```python
from build123d import *

# Parameters (mm, degrees)
SKETCH_1_W         = 25.5
SKETCH_1_H         = 25
EXTRUDE_1_DEPTH    = 4
SKETCH_6_W         = 25.5
SKETCH_6_H         = 7
EXTRUDE_2_DEPTH    = 9
HOLE_WIZARD_M3_1_D = 2.5
HOLE_WIZARD_M4_3_D = 3.3
FILLET_1_R         = 1


with BuildPart() as part:
    # 草图1 → 凸台-拉伸1 (new body)
    with BuildSketch(Plane(origin=(0, 0, 0), x_dir=(1, 0, 0), z_dir=(0, 1, 0))):
        Rectangle(SKETCH_1_W, SKETCH_1_H)
    extrude(amount=EXTRUDE_1_DEPTH)

    # 草图6 → 凸台-拉伸2 (add)
    with BuildSketch(Plane(origin=(0, 4, 0), x_dir=(1, 0, 0), z_dir=(0, 1, 0))):
        with Locations((0, 9)):
            Rectangle(SKETCH_6_W, SKETCH_6_H)
        with Locations((0, -9)):
            Rectangle(SKETCH_6_W, SKETCH_6_H)
    extrude(amount=EXTRUDE_2_DEPTH)

    # M3 螺纹孔1 (through all)
    with Locations(Plane(origin=(6.35, 0, 0), x_dir=(0, 0, -1), z_dir=(0, -1, 0))):
        with Locations((0, 0), (0, -12.7)):
            Hole(HOLE_WIZARD_M3_1_D / 2)

    # M4 螺纹孔3 (through all)
    with Locations(Plane(origin=(7.5, 0, 8.5), x_dir=(0, 0, -1), z_dir=(0, -1, 0))):
        with Locations((0, 0), (0, -15), (17, -15), (17, 0)):
            Hole(HOLE_WIZARD_M4_3_D / 2)

    # 圆角1
    fillet_1_edges = [part.edges().sort_by_distance(p)[0] for p in [
        (0, 4, -5.5),
        (0, 13, -12.5),
        (0, 4, 5.5),
        (0, 13, 12.5),
        (0, 0, 12.5),
        (0, 0, -12.5),
    ]]
    fillet(fillet_1_edges, radius=FILLET_1_R)


solid = part.part
```
Check sheet for the modelled part. Datum: model origin and axes. Units: mm. A direction names the side the tool comes from. Coordinates: 2 decimals unless noted, no trailing zeros. Write each loop counter-clockwise with the first axis right and the second up, starting at its lowest first coordinate (ties: lowest second). Pieces come first, ordered by that corner, then holes. Notation, with made-up numbers: M -37,-10 L -3,-10 A26 cw -3,25 Z; hole C 17,46 d5. An arc over 180 degrees is marked long. Write item = value, one per line. Start each with the question number.
1. Sectioned sample at C-C (x = -6.35). Record the cut outline in (y, z), then the cut area to 3 significant figures.
2. Sectioned sample at D-D (x = 0). Record the cut outline in (y, z), then the cut area to 3 significant figures.
3. Thickness scan on probe 1 along X at (y, z) = (10, 8.5); probe 2 along X at (y, z) = (10.25, -9.25); probe 3 along Z at (x, y) = (1, 6). Record the ranges inside material, lowest first.
4. Sectioned sample at A-A (y = 8.5). Record the cut outline in (x, z).
5. Go/stop test with flat-tipped pins: pin 1 (2.5 mm diameter, centred on x = -2, z = -2, fed in from +Y); pin 2 (3 mm diameter, centred on x = 6.35, z = 0, fed in from -Y). Record where each tip stops, or that it passes through.
6. Mould release check, pull along X, two halves, no side actions. Record for faces 1 (the flat face through (-12.75, 3.5, 0.2)), 2 (the cylindrical face through (-5.11, 2.03, -0.16)), 3 (the cylindrical face through (-7.43, 6.59, -10.15)), 4 (the flat face through (0, 6, 12.5)): pulls with the +X half, pulls with the -X half, needs draft (parallel to the pull), parting line crosses it, or undercut.
7. Sectioned sample at B-B (z = -0.75). Record the cut outline in (x, y), then the cut area to 3 significant figures.
8. Tool access check on faces 5 (the cylindrical face through (7.59, 2.03, -0.16)), 6 (the flat face through (0, 9, 5.5)). Record the directions out of +Z, -Z, +X, -X, +Y, -Y that give a thin tool (end or side, any length) a straight path to the whole face; none if there is none.
The answers:
q1.outline = M 0,-11.5 A1 ccw 1,-12.5 L 12,-12.5 A1 ccw 13,-11.5 L 13,-9.68 L 0,-9.68 Z; M 0,-7.32 L 13,-7.32 L 13,-5.5 L 5,-5.5 A1 cw 4,-4.5 L 4,-1.25 L 0,-1.25 Z; M 0,1.25 L 4,1.25 L 4,4.5 A1 cw 5,5.5 L 13,5.5 L 13,7.32 L 0,7.32 Z; M 0,9.68 L 13,9.68 L 13,11.5 A1 ccw 12,12.5 L 1,12.5 A1 ccw 0,11.5 Z
q1.area = 154 mm²
q2.outline = M 0,-11.5 A1 ccw 1,-12.5 L 12,-12.5 A1 ccw 13,-11.5 L 13,-5.5 L 5,-5.5 A1 cw 4,-4.5 L 4,4.5 A1 cw 5,5.5 L 13,5.5 L 13,11.5 A1 ccw 12,12.5 L 1,12.5 A1 ccw 0,11.5 Z
q2.area = 226 mm²
q3.probe_1 = -12.75 to -9.15, -5.85 to 5.85, 9.15 to 12.75
q3.probe_2 = -12.75 to -8.97, -6.03 to 6.03, 8.97 to 12.75
q3.probe_3 = -12.5 to -5.5, 5.5 to 12.5
q4.outline = M -12.75,-12.5 L 12.75,-12.5 L 12.75,-5.5 L -12.75,-5.5 Z; M -12.75,5.5 L 12.75,5.5 L 12.75,12.5 L -12.75,12.5 Z; hole C -7.5,-8.5 d3.3; hole C -7.5,8.5 d3.3; hole C 7.5,-8.5 d3.3; hole C 7.5,8.5 d3.3
q5.pin_1 = 4
q5.pin_2 = 0
q6.face_1 = pulls with the -X half
q6.face_2 = undercut
q6.face_3 = undercut
q6.face_4 = needs draft
q7.outline = M -12.75,0 L -7.35,0 L -7.35,4 L -12.75,4 Z; M -5.35,0 L 5.35,0 L 5.35,4 L -5.35,4 Z; M 7.35,0 L 12.75,0 L 12.75,4 L 7.35,4 Z
q7.area = 86.0 mm²
q8.face_5 = +Y, -Y
q8.face_6 = +X, -X, +Y
